```python
from build123d import *

# Parameters (mm, degrees)
SKETCH_1_R      = 1.5
EXTRUDE_1_DEPTH = 6


with BuildPart() as part:
    # 草图1 → 凸台-拉伸1 (new body)
    with BuildSketch(Plane(origin=(0, 0, 0), x_dir=(1, 0, 0), z_dir=(0, 1, 0))):
        Polygon((-162.5, 65), (2.497803149, 65), (2.497803149, 61.454616174), (130.785768407, 61.454616174), (130.785768407, 65), (162.5, 65), (162.5, -65), (-162.5, -65), align=None)
        with Locations(Location((-152.5, 55, 0), (0, 0, 270))):
            Circle(SKETCH_1_R, mode=Mode.SUBTRACT)
        with Locations(Location((-152.5, -55, 0), (0, 0, 270))):
            Circle(SKETCH_1_R, mode=Mode.SUBTRACT)
        with Locations(Location((-92.5, 55, 0), (0, 0, 270))):
            Circle(SKETCH_1_R, mode=Mode.SUBTRACT)
        with Locations(Location((-32.5, 55, 0), (0, 0, 270))):
            Circle(SKETCH_1_R, mode=Mode.SUBTRACT)
        with Locations(Location((27.5, 55, 0), (0, 0, 270))):
            Circle(SKETCH_1_R, mode=Mode.SUBTRACT)
        with Locations(Location((87.5, 55, 0), (0, 0, 270))):
            Circle(SKETCH_1_R, mode=Mode.SUBTRACT)
        with Locations(Location((147.5, 55, 0), (0, 0, 270))):
            Circle(SKETCH_1_R, mode=Mode.SUBTRACT)
        with Locations(Location((-92.5, -55, 0), (0, 0, 270))):
            Circle(SKETCH_1_R, mode=Mode.SUBTRACT)
        with Locations(Location((-32.5, -55, 0), (0, 0, 270))):
            Circle(SKETCH_1_R, mode=Mode.SUBTRACT)
        with Locations(Location((27.5, -55, 0), (0, 0, 270))):
            Circle(SKETCH_1_R, mode=Mode.SUBTRACT)
        with Locations(Location((87.5, -55, 0), (0, 0, 270))):
            Circle(SKETCH_1_R, mode=Mode.SUBTRACT)
        with Locations(Location((147.5, -55, 0), (0, 0, 270))):
            Circle(SKETCH_1_R, mode=Mode.SUBTRACT)
        with Locations(Location((-152.5, 0, 0), (0, 0, 270))):
            Circle(SKETCH_1_R, mode=Mode.SUBTRACT)
    extrude(amount=EXTRUDE_1_DEPTH)


solid = part.part
```
The model under review builds one solid part; all positions refer to its coordinate system, in mm. Round coordinates to 2 decimals unless told otherwise and drop trailing zeros. Answer as CSV lines item,"result". Start each with the question number.
(1) To check wall thickness, follow line 1 (Z direction, x = -152.5, y = 2.3); line 2 (Z direction, x = 88.5, y = 5.8); line 3 (Z direction, x = 106, y = 4.8). State the ranges of each line that lie inside material, in increasing order.
(2) Draft analysis for pull direction X (two halves, no side actions). For faces 1 (the flat face through (66, 3, -61.455)), 2 (the flat face through (146, 3, -65)), 3 (the flat face through (162.5, 3, -1)), state which applies: pulls with the +X half, pulls with the -X half, needs draft (parallel to the pull), parting line crosses it, or undercut.
(3) For pin 1 Ø1 at (x, y) = (91.5, 1) entering from -Z, flat-tipped, find the tip position at first contact; note if it passes through.
Worked answers:
1,line 1,"-65 to -56.5, -53.5 to -1.5, 1.5 to 53.5, 56.5 to 65"
1,line 2,"-61.45 to -56.12, -53.88 to 53.88, 56.12 to 65"
1,line 3,"-61.45 to 65"
2,face 1,"undercut"
2,face 2,"needs draft"
2,face 3,"pulls with the +X half"
3,pin 1,"z = -61.45"
